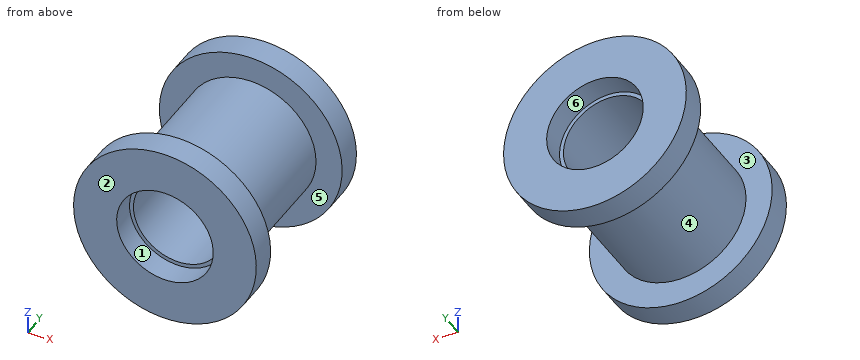
from build123d import *

# Parameters (mm, degrees)
SKETCH_1_R          = 35
EXTRUDE_1_DEPTH     = 10
SKETCH_5_R          = 25
EXTRUDE_2_DEPTH     = 50
SKETCH_6_R          = 35
EXTRUDE_3_DEPTH     = 10
SKETCH_7_R          = 18.5
CUT_EXTRUDE_1_DEPTH = 9
SKETCH_8_R          = 17
CUT_EXTRUDE_2_DEPTH = 52
SKETCH_9_R          = 18.5
CUT_EXTRUDE_3_DEPTH = 79.555712714


with BuildPart() as part:
    # 草图1 → 凸台-拉伸1 (new body)
    with BuildSketch(Plane(origin=(0, 0, 0), x_dir=(1, 0, 0), z_dir=(0, 1, 0))):
        with Locations(Location((0, 0, 0), (0, 0, 270))):
            Circle(SKETCH_1_R)
    extrude(amount=EXTRUDE_1_DEPTH)

    # 草图5 → 凸台-拉伸2 (add)
    with BuildSketch(Plane(origin=(0, 10, 0), x_dir=(1, 0, 0), z_dir=(0, 1, 0))):
        with Locations(Location((0, 0, 0), (0, 0, 270))):
            Circle(SKETCH_5_R)
    extrude(amount=EXTRUDE_2_DEPTH)

    # 草图6 → 凸台-拉伸3 (add)
    with BuildSketch(Plane(origin=(0, 60, 0), x_dir=(1, 0, 0), z_dir=(0, 1, 0))):
        with Locations(Location((0, 0, 0), (0, 0, 270))):
            Circle(SKETCH_6_R)
    extrude(amount=EXTRUDE_3_DEPTH)

    # 草图7 → 切除-拉伸1 (cut)
    with BuildSketch(Plane(origin=(0, 70, 0), x_dir=(1, 0, 0), z_dir=(0, 1, 0))):
        with Locations(Location((0, 0, 0), (0, 0, 270))):
            Circle(SKETCH_7_R)
    extrude(amount=-CUT_EXTRUDE_1_DEPTH, mode=Mode.SUBTRACT)

    # 草图8 → 切除-拉伸2 (cut)
    with BuildSketch(Plane(origin=(0, 61, 0), x_dir=(1, 0, 0), z_dir=(0, 1, 0))):
        with Locations(Location((0, 0, 0), (0, 0, 270))):
            Circle(SKETCH_8_R)
    extrude(amount=-CUT_EXTRUDE_2_DEPTH, mode=Mode.SUBTRACT)

    # 草图9 → 切除-拉伸3 (cut, through all)
    with BuildSketch(Plane(origin=(0, 9, 0), x_dir=(1, 0, 0), z_dir=(0, 1, 0))):
        with Locations(Location((0, 0, 0), (0, 0, 270))):
            Circle(SKETCH_9_R)
    extrude(amount=-CUT_EXTRUDE_3_DEPTH, mode=Mode.SUBTRACT)


solid = part.part
Work out the finished part from the listing and answer in its coordinate system (mm). Face numbers are marked on the shaded views. A direction names the side the tool comes from. Coordinates: 2 decimals unless noted, no trailing zeros. Write each loop counter-clockwise with the first axis right and the second up, starting at its lowest first coordinate (ties: lowest second). Pieces come first, ordered by that corner, then holes.
1. The part is cut by section C-C, the plane y = 26. Write down the section's boundary in (x, z).
Results list:
outline: circle Ø50 at (0, 0); hole circle Ø34 at (0, 0)
2. The part is cut by section D-D, the plane z = -20. Write down the section's boundary in (x, y).
Results list:
outline: (-28.72, 0) - (28.72, 0) - (28.72, 10) - (15, 10) - (15, 60) - (28.72, 60) - (28.72, 70) - (-28.72, 70) - (-28.72, 60) - (-15, 60) - (-15, 10) - (-28.72, 10) - close
3. Consider line 1 along X through (y, z) = (48.5, 0); line 2 along Y through (x, z) = (9, 23.5); line 3 along X through (y, z) = (4, 0). Determine where each line is inside the solid, lowest interval first.
Results list:
line 1: x = -25 to -17, 17 to 25
line 2: y = 0 to 10, 60 to 70
line 3: x = -35 to -18.5, 18.5 to 35
4. Flat-ended cylindrical pins translate along their axes: pin 1 (5 mm diameter, centred on y = 59, z = -21, fed in from +X); pin 2 (3 mm diameter, centred on y = 32.5, z = -22.5, fed in from +X); pin 3 (12 mm diameter, centred on y = 40, z = 19.5, fed in from +X); pin 4 (3 mm diameter, centred on x = 13.5, z = 5, fed in from -Y). Find the tip coordinate at first contact, or state that the pin passes through.
Results list:
pin 1: stops at x = 29.58
pin 2: stops at x = 13.56
pin 3: stops at x = 21.04
pin 4: passes through
5. The part is cut by section B-B, the plane z = 0. Write down the section's boundary in (x, y), and give its area (3 significant figures).
Results list:
outline: (-35, 0) - (-18.5, 0) - (-18.5, 9) - (-17, 9) - (-17, 61) - (-18.5, 61) - (-18.5, 70) - (-35, 70) - (-35, 60) - (-25, 60) - (-25, 10) - (-35, 10) - close; (17, 9) - (18.5, 9) - (18.5, 0) - (35, 0) - (35, 10) - (25, 10) - (25, 60) - (35, 60) - (35, 70) - (18.5, 70) - (18.5, 61) - (17, 61) - close
area: 1,470 mm2
6. The part is cut by section A-A, the plane x = 0. Write down the section's boundary in (y, z), and give its area (3 significant figures).
Results list:
outline: (0, -35) - (10, -35) - (10, -25) - (60, -25) - (60, -35) - (70, -35) - (70, -18.5) - (61, -18.5) - (61, -17) - (9, -17) - (9, -18.5) - (0, -18.5) - close; (0, 18.5) - (9, 18.5) - (9, 17) - (61, 17) - (61, 18.5) - (70, 18.5) - (70, 35) - (60, 35) - (60, 25) - (10, 25) - (10, 35) - (0, 35) - close
area: 1,470 mm2
7. For the marked faces 1, 2 and 3, determine the directions among +Z, -Z, +X, -X, +Y, -Y from which every point of the face is accessible in a straight line to the end or side of a thin tool.
Results list:
face 1: -Y
face 2: +Z, -Z, +X, -X, -Y
face 3: none
8. For a pull along X with two mould halves and no side action, classify the marked faces 4, 5 and 6 as +X half, -X half, draft (parallel to the pull), parting line (faces both ways), or undercut.
Results list:
face 4: parting line
face 5: draft
face 6: undercut
